Source: CAD feature listing. Evaluate the final solid. Frame: model axes, mm. A direction names the side the tool comes from. Give positions to 0.01 mm unless a question says otherwise; leave off trailing zeros. Order: outer loops, then holes, each group sorted by start corner. A loop starts at its lowest first (then second) coordinate and runs counter-clockwise, first axis right, second up. Notation, with made-up numbers: M 86,75 L 100,75 A23 ccw 100,112 Z; hole C 58.5,-14 d5. An arc over 180 degrees is marked long. Use CSV: the item, a comma, the result in double quotes. Start each with the question number.
1. Section query C-C, the plane y = 25.5. Return the cut outline in (x, z) (3 decimals), plus the area to 3 significant figures.
2. Pin query (flat end, axial travel): P1, Ø0.8, axis at y = 25.5, z = 12, coming from the -X side; P2, Ø0.8, axis at x = 0, y = 24.5, coming from the +Z side (3 decimals); P3, Ø4, axis at x = -9, z = -8.5, coming from the -Y side. Return the tip coordinate at first contact, or that it passes through.
3. Reachability of faces 1 (the flat face through (-17, 0, 7)), 2 (the flat face through (-0.5, 23.5, 12.4)), 3 (the cylindrical face through (-12.122, 22.957, -0.26)) from +Z, -Z, +X, -X, +Y, -Y: full face, straight path, thin tool, end or side. Return the list, or none.
4. Section query D-D, the plane y = 12.5. Return the cut outline in (x, z).
5. Section query A-A, the plane z = 0. Return the cut outline in (x, y) (3 decimals), plus the area to 3 significant figures.
6. Line query: line 1 along X through (y, z) = (9.5, 0); line 2 along Y through (x, z) = (-7.5, 16.5); line 3 along Y through (x, z) = (11, -2). Output: solid intervals per line, ascending. Write a range as [from, to].
7. Section query B-B, the plane x = 0. Return the cut outline in (y, z) (3 decimals), plus the area to 3 significant figures.
from build123d import *

# Parameters (mm, degrees)
SKETCH2_R               = 18.85
BOSS_EXTRUDE1_DEPTH     = 15
SKETCH4_R               = 17.85
CUT_EXTRUDE2_DEPTH      = 13
SKETCH5_R               = 13.125
BOSS_EXTRUDE2_DEPTH     = 12
SKETCH6_R               = 12.125
CUT_EXTRUDE3_DEPTH      = 38.942654098
CUT_EXTRUDE5_DEPTH      = 12
CUT_EXTRUDE5_DEPTH_BACK = 38.942654098
SKETCH11_W              = 1
SKETCH11_H              = 5
CUT_EXTRUDE7_DEPTH      = 31.711683494
BOSS_EXTRUDE4_START     = -5.8
SKETCH12_R              = 17.85
SKETCH12_R_2            = 12.125
BOSS_EXTRUDE4_DEPTH     = 5.8
FILLET3_R               = 5.8


with BuildPart() as part:
    # Sketch2 → Boss-Extrude1 (new body)
    with BuildSketch(Plane(origin=(0, 0, 0), x_dir=(1, 0, 0), z_dir=(0, 1, 0))):
        with Locations(Location((0, 0, 0), (0, 0, 270))):
            Circle(SKETCH2_R)
    extrude(amount=BOSS_EXTRUDE1_DEPTH)

    # Sketch4 → Cut-Extrude2 (cut)
    with BuildSketch(Plane(origin=(0, 0, 0), x_dir=(-1, 0, 0), z_dir=(0, -1, 0))):
        with Locations(Location((0, 0, 0), (0, 0, 90))):
            Circle(SKETCH4_R)
    extrude(amount=-CUT_EXTRUDE2_DEPTH, mode=Mode.SUBTRACT)

    # Sketch5 → Boss-Extrude2 (add)
    with BuildSketch(Plane(origin=(0, 15, 0), x_dir=(1, 0, 0), z_dir=(0, 1, 0))):
        with Locations(Location((0, 0, 0), (0, 0, 270))):
            Circle(SKETCH5_R)
    extrude(amount=BOSS_EXTRUDE2_DEPTH)

    # Sketch6 → Cut-Extrude3 (cut, through all)
    with BuildSketch(Plane(origin=(0, 27, 0), x_dir=(1, 0, 0), z_dir=(0, 1, 0))):
        with Locations(Location((0, 0, 0), (0, 0, 270))):
            Circle(SKETCH6_R)
    extrude(amount=-CUT_EXTRUDE3_DEPTH, mode=Mode.SUBTRACT)

    # Sketch7 → Cut-Extrude5 (cut, two sides: drawn at the far end of the back side and taken through both)
    with BuildSketch(Plane(origin=(0, 27, 0), x_dir=(1, 0, 0), z_dir=(0, 1, 0)).offset(-CUT_EXTRUDE5_DEPTH_BACK)):
        with BuildLine():
            ThreePointArc((-0.5, 12.114686335), (-0.25005318, 12.12242131), (0, 12.125))
            Line((0, 12.125), (0, 12.625))
            Line((0, 12.625), (-0.5, 12.625))
            Line((-0.5, 12.625), (-0.5, 12.114686335))
        make_face()
        with BuildLine():
            Line((0, 12.625), (0, 12.125))
            ThreePointArc((0, 12.125), (0.25005318, 12.12242131), (0.5, 12.114686335))
            Line((0.5, 12.114686335), (0.5, 12.625))
            Line((0.5, 12.625), (0, 12.625))
        make_face()
        with BuildLine():
            Line((0, -12.625), (0, -12.125))
            ThreePointArc((0, -12.125), (-0.25005318, -12.12242131), (-0.5, -12.114686335))
            Line((-0.5, -12.114686335), (-0.5, -12.625))
            Line((-0.5, -12.625), (0, -12.625))
        make_face()
        with BuildLine():
            ThreePointArc((0.5, -12.114686335), (0.25005318, -12.12242131), (0, -12.125))
            Line((0, -12.125), (0, -12.625))
            Line((0, -12.625), (0.5, -12.625))
            Line((0.5, -12.625), (0.5, -12.114686335))
        make_face()
    extrude(amount=CUT_EXTRUDE5_DEPTH + CUT_EXTRUDE5_DEPTH_BACK, mode=Mode.SUBTRACT)

    # Sketch8 → Revolve3 (revolve)
    with BuildSketch(Plane(origin=(0, 27, 0), x_dir=(0, 0, 1), z_dir=(-1, 0, 0))):
        with BuildLine():
            Line((-11.125, 1), (-11.125, 1.25))
            Line((-11.125, 1.25), (-11.875, 1.25))
            ThreePointArc((-11.875, 1.25), (-12.758883476, 0.883883476), (-13.125, 0))
            Line((-13.125, 0), (-12.125, 0))
            ThreePointArc((-12.125, 0), (-11.832106781, 0.707106781), (-11.125, 1))
        make_face()
    revolve(axis=Axis((0, 13, 0), (0, 1, 0)))

    # Sketch11 → Cut-Extrude7 (cut, through all)
    with BuildSketch(Plane.XZ.offset(-13)):
        with Locations((0, -10.125)):
            Rectangle(SKETCH11_W, SKETCH11_H)
        with Locations((0, 10.125)):
            Rectangle(SKETCH11_W, SKETCH11_H)
    extrude(amount=-CUT_EXTRUDE7_DEPTH, mode=Mode.SUBTRACT)

    # Sketch12 → Boss-Extrude4 (add)
    with BuildSketch(Plane(origin=(0, 13, 0), x_dir=(-1, 0, 0), z_dir=(0, -1, 0)).offset(BOSS_EXTRUDE4_START)):
        with Locations(Location((0, 0, 0), (0, 0, 90))):
            Circle(SKETCH12_R)
        with Locations(Location((0, 0, 0), (0, 0, 267.636617298))):
            Circle(SKETCH12_R_2, mode=Mode.SUBTRACT)
    extrude(amount=BOSS_EXTRUDE4_DEPTH)

    # Fillet3
    # the kernel refuses this fillet: 5.8 mm, written as the material it takes off along each edge
    with BuildSketch(Plane(origin=(0, 13, 0), x_dir=(0.04123711340209573, 0, 0.999149388469143), z_dir=(-0.999149388469143, 0, 0.04123711340209573))) as fillet3_piece_1_section:
        with BuildLine():
            CenterArc((12.125 + FILLET3_R, FILLET3_R), FILLET3_R, 180, 90)
            Line((12.125 + FILLET3_R, 0), (12.125, 0))
            Line((12.125, 0), (12.125, FILLET3_R))
        make_face()
    fillet3_piece_1 = revolve(axis=Axis((0, 13, 0), (0, 1, 0)), mode=Mode.PRIVATE)
    fillet3_piece_1 = fillet3_piece_1 & Plane(origin=(0, 14.662321343, 0), x_dir=(0, 0, -1), z_dir=(0, -1, 0)) * Cylinder(17.85, 72, mode=Mode.PRIVATE)
    add(fillet3_piece_1, mode=Mode.SUBTRACT)


solid = part.part
Result set:
1,outline,"C 0,0 d26.25; hole M -0.5,-12.625 L 0.5,-12.625 L 0.5,-12.115 A12.125 ccw 0.5,12.115 L 0.5,12.625 L -0.5,12.625 L -0.5,12.115 A12.125 ccw -0.5,-12.115 Z"
1,area,"78.3 mm2"
2,P1,"x = -6.14"
2,P2,"z = 13.125"
2,P3,"y = 14.21"
3,face 1,"+Z, -Z, +X, -X, -Y"
3,face 2,"+Y"
3,face 3,"-Y"
4,outline,"C 0,0 d37.7; hole C 0,0 d35.7"
5,outline,"M -18.85,0 L -17.85,0 L -17.85,13 A5.8 ccw -12.125,18.8 L -12.125,27 A1 cw -11.125,28 L -11.125,28.25 L -11.875,28.25 A1.25 ccw -13.125,27 L -13.125,18.8 L -17.85,18.8 L -17.85,15 L -18.85,15 Z; M 11.125,28 A1 cw 12.125,27 L 12.125,18.8 A5.8 ccw 17.85,13 L 17.85,0 L 18.85,0 L 18.85,15 L 17.85,15 L 17.85,18.8 L 13.125,18.8 L 13.125,27 A1.25 ccw 11.875,28.25 L 11.125,28.25 Z"
5,area,"101 mm2"
6,line 1,"[-18.85, -17.85], [17.85, 18.85]"
6,line 2,"[0, 15]"
6,line 3,"[28, 28.25]"
7,outline,"M 0,-18.85 L 15,-18.85 L 15,-17.85 L 18.8,-17.85 L 18.8,-13.125 L 27,-13.125 A1.25 ccw 28,-12.625 L 18.8,-12.625 L 18.8,-12.125 A5.8 ccw 13,-17.85 L 0,-17.85 Z; M 0,17.85 L 13,17.85 A5.8 ccw 18.8,12.125 L 18.8,12.625 L 28,12.625 A1.25 ccw 27,13.125 L 18.8,13.125 L 18.8,17.85 L 15,17.85 L 15,18.85 L 0,18.85 Z"
7,area,"90.9 mm2"
